from build123d import *

# Parameters (mm, degrees)
F2_R     = 1.75
F3_DEPTH = 7.5
F4_SIZE  = 2


with BuildPart() as f1:
    # F0 (on Front) → F1 (revolve)
    with BuildSketch(Plane.XZ):
        Polygon((0, 8), (0, 0), (7.5, 0), (7.5, 1.5), (3, 1.5), (3, 8), align=None)
    revolve(axis=Axis((0, 0, 7.429687), (0, 0, 1)))

    # F2 (on face) → F3 (cut)
    with BuildSketch(Plane.XY.offset(8)):
        Circle(F2_R)
    extrude(amount=-F3_DEPTH, mode=Mode.SUBTRACT)

    # F4
    f4_edges = [f1.edges().sort_by_distance(p)[0] for p in [
        (-3, 0, 1.5),
    ]]
    chamfer(f4_edges, length=F4_SIZE)


solid = f1.part
Could you check a few things on this model? Use its own coordinates, in mm. A direction names the side the tool comes from. Give positions to 0.01 mm unless a question says otherwise; leave off trailing zeros. Write each loop counter-clockwise with the first axis right and the second up, starting at its lowest first coordinate (ties: lowest second). Pieces come first, ordered by that corner, then holes. Notation, with made-up numbers: (-5, -26) -> (6, -26) arc R21 ccw to (6, 0) -> close; hole circle Ø3 at (29.5, 72). An arc over 180 degrees is marked (long way). Answer as CSV lines item,"result". Start each with the question number.
(1) If we section it at C-C, the plane z = 1: Write out the boundary of the cut face in (x, y), and give its area (3 significant figures).
(2) Which directions (+Z, -Z, +X, -X, +Y, -Y) give clear straight access to the entire face, cutting with the end or side of a thin tool? Please do faces 4 (the face through (0, -2, 8)), 5 (the face through (0, 0, 0.5)).
(3) If we section it at A-A, the plane y = 0: Write out the boundary of the cut face in (x, z).
(4) If we section it at D-D, the plane z = 2: Write out the boundary of the cut face in (x, y).
(5) If we mould it in two halves opening along Y, with no side actions, what happens to faces 1 (the face through (1.617, -0.67, 4.302)), 2 (the face through (0, 0, 0)), 3 (the face through (-3, 0, 6))? For each: +Y half, -Y half, draft (parallel to the pull), parting line (faces both ways), or undercut.
(6) Please list where these lines run through material, in increasing order: line 1 (Y direction, x = 0, z = 4.5); line 2 (Z direction, x = 4.75, y = -4.25); line 3 (X direction, y = -0.5, z = 6.25).
(7) I'm going to push flat-ended pins straight in: pin 1 Ø5 at (x, y) = (2, -0.5) entering from -Z; pin 2 Ø2 at (x, y) = (1, 5.5) entering from +Z; pin 3 Ø3 at (x, z) = (-0.5, 5.5) entering from -Y. Where does each tip first touch, or does it pass through?
Answer list:
1,outline,"circle Ø15 at (0, 0); hole circle Ø3.5 at (0, 0)"
1,area,"167 mm^2"
2,face 4,"+Z, +X, -X, +Y, -Y"
2,face 5,"+Z"
3,outline,"(-7.5, 0) -> (7.5, 0) -> (7.5, 1.5) -> (5, 1.5) -> (3, 3.5) -> (3, 8) -> (1.75, 8) -> (1.75, 0.5) -> (-1.75, 0.5) -> (-1.75, 8) -> (-3, 8) -> (-3, 3.5) -> (-5, 1.5) -> (-7.5, 1.5) -> close"
4,outline,"circle Ø9 at (0, 0); hole circle Ø3.5 at (0, 0)"
5,face 1,"undercut"
5,face 2,"draft"
5,face 3,"parting line"
6,line 1,"-3 to -1.75, 1.75 to 3"
6,line 2,"0 to 1.5"
6,line 3,"-2.96 to -1.68, 1.68 to 2.96"
7,pin 1,"z = 0"
7,pin 2,"z = 1.91"
7,pin 3,"y = -3"
